from build123d import *

# Parameters (mm, degrees)
F0_R     = 16.5
F1_DEPTH = 8
F2_R     = 1.05
F3_DEPTH = 2.5
F4_R     = 1
F5_DEPTH = 2.5
F7_DEPTH = 25


with BuildPart() as f1:
    # F0 (on Top) → F1 (new body)
    with BuildSketch(Plane.XY):
        Circle(F0_R)
    extrude(amount=F1_DEPTH)

    # F2 (on face) → F3 (cut)
    with BuildSketch(Plane(origin=(0, 0, 0), x_dir=(1, 0, 0), z_dir=(0, 0, -1))):
        with Locations((0, 15.05)):
            Circle(F2_R)
        with Locations((15, 0.05)):
            Circle(F2_R)
        with Locations((0, -14.95)):
            Circle(F2_R)
    extrude(amount=-F3_DEPTH, mode=Mode.SUBTRACT)

    # F4 (on face) → F5 (join)
    with BuildSketch(Plane.XY.offset(8)):
        with Locations((0, 15)):
            Circle(F4_R)
        with Locations((15, 0)):
            Circle(F4_R)
        with Locations((0, -15)):
            Circle(F4_R)
    extrude(amount=F5_DEPTH)

    # F6 (on face) → F7 (cut)
    with BuildSketch(Plane.XY.offset(8)):
        Polygon((-14, 5.79899), (-14, -5.79899), (-10, -4.142136), (-10, 4.142136), align=None)
        Polygon((4.142136, 10), (5.79899, 14), (0, 14), (-5.79899, 14), (-4.142136, 10), align=None)
        Polygon((10, -4.142136), (14, -5.79899), (14, 0), (14, 5.79899), (10, 4.142136), align=None)
        Polygon((-9, -3.727922), (-3.727922, -9), (-2.485281, -6), (-6, -2.485281), align=None)
        Polygon((3.727922, -9), (9, -3.727922), (6, -2.485281), (2.485281, -6), align=None)
        Polygon((-2.485281, 6), (-3.727922, 9), (-9, 3.727922), (-6, 2.485281), align=None)
        Polygon((6, 2.485281), (9, 3.727922), (3.727922, 9), (2.485281, 6), align=None)
        Polygon((-5, -2.071068), (0, 0), (-5, 2.071068), align=None)
    extrude(amount=-F7_DEPTH, mode=Mode.SUBTRACT)


solid = f1.part
Geometry: final body of the model. Coordinates: model frame, mm. A direction names the side the tool comes from. Give positions to 0.01 mm unless a question says otherwise; leave off trailing zeros. Loops run counter-clockwise (first coordinate to the right, second up) from the corner with the lowest first, then second, coordinate; pieces in that order, holes last. Notation, with made-up numbers: M 46.5,37 L 101.5,37 A9 cw 101.5,54 Z; hole C 81,-20.5 d3. An arc over 180 degrees is marked long. Put each result on its own line as item: value. Start each with the question number.
1) Pull-direction query (X, two-part tool) for faces 4 (the cylindrical face through (16, 0, 9)), 5 (the flat face through (-4.267, 4.218, 4.056)), 6 (the flat face through (0, -3, 8)); classes: pulls with the +X half, pulls with the -X half, needs draft (parallel to the pull), parting line crosses it, or undercut.
2) Access query for faces 1 (the flat face through (10, 0, 4)), 2 (the cylindrical face through (16.05, -0.01, 1.23)), 3 (the flat face through (0, -15, 10.5)). Directions: +Z, -Z, +X, -X, +Y, -Y. A direction counts if a zero-diameter tool reaches every point of the face in a straight line with its end or side. Return the directions, or none.
3) Cut plane B-B (x = 12). Output: boundary loops of the cut face in (y, z), then the cut area to 3 significant figures.
4) Contact query for flat-ended pins moving along their axis: pin 1 (6 mm diameter, centred on y = -9.5, z = 5, fed in from -X); pin 2 (1 mm diameter, centred on x = -8, z = 4.5, fed in from -Y); pin 3 (1.6 mm diameter, centred on x = 15, y = 0, fed in from -Z). Output: stop coordinate, or through.
5) Ray query, line 1 along X through (y, z) = (-0.05, 1.8); line 2 along X through (y, z) = (0.5, 7.5); line 3 along Y through (x, z) = (-3, 2). Return the intervals inside material, ascending.
6) Cut plane A-A (z = 3). Give the number of separate pieces and of enclosed holes in the cut face, then the cut area to 3 significant figures.
7) Cut plane D-D (y = 3). Output: boundary loops of the cut face in (x, z), then the cut area to 3 significant figures.
8) Cut plane C-C (y = 11.5). Output: boundary loops of the cut face in (x, z), then the cut area to 3 significant figures.
Verdict:
1. face 4: parting line crosses it
1. face 5: undercut
1. face 6: needs draft
2. face 1: +Z, -Z
2. face 2: -Z
2. face 3: +Z, +X, -X, +Y, -Y
3. outline: M -11.32,0 L -4.97,0 L -4.97,8 L -11.32,8 Z; M 4.97,0 L 11.32,0 L 11.32,8 L 4.97,8 Z
3. area: 102 mm2
4. pin 1: x = -15.17
4. pin 2: y = -14.7
4. pin 3: z = 2.5
5. line 1: -16.5 to -14, -10 to -5, -0.12 to 10, 16.05 to 16.5
5. line 2: -16.49 to -14, -10 to -5, -1.21 to 10, 14 to 16.49
5. line 3: -16.22 to -7.24, -5.49 to -1.24, 1.24 to 5.49, 7.24 to 10, 14 to 16.22
6. separate pieces: 1
6. enclosed holes: 8
6. area: 651 mm2
7. outline: M -16.22,0 L -14,0 L -14,8 L -16.22,8 Z; M -10,0 L -7.24,0 L -7.24,8 L -10,8 Z; M -5.49,0 L 5.49,0 L 5.49,8 L -5.49,8 Z; M 7.24,0 L 10,0 L 10,8 L 7.24,8 Z; M 14,0 L 16.22,0 L 16.22,8 L 14,8 Z
7. area: 167 mm2
8. outline: M -11.83,0 L -4.76,0 L -4.76,8 L -11.83,8 Z; M 4.76,0 L 11.83,0 L 11.83,8 L 4.76,8 Z
8. area: 113 mm2
